Design review of the part built by this model. Coordinates are the model's own, in mm. A direction names the side the tool comes from. Round coordinates to 2 decimals unless told otherwise and drop trailing zeros. Write each loop counter-clockwise with the first axis right and the second up, starting at its lowest first coordinate (ties: lowest second). Pieces come first, ordered by that corner, then holes. Notation, with made-up numbers: (44.25, 16.5) -> (97.25, 16.5) arc R20 cw to (97.25, 20.5) -> close; hole circle Ø10 at (4, 86.25). An arc over 180 degrees is marked (long way). Write item = value, one per line. Start each with the question number.
Item 1: Add section A-A, the plane z = -13.5. State the section outline as (x, y) points, then the cut area to 3 significant figures.
Item 2: For pin 1 Ø17 at (x, z) = (123.5, -13.5) entering from -Y; pin 2 Ø2 at (x, z) = (120, -16.5) entering from -Y; pin 3 Ø4 at (x, z) = (121.5, -12.5) entering from -Y, all flat-tipped, find the tip position at first contact; note any pin that passes through.
Item 3: Add section C-C, the plane z = -3.5. State the section outline as (x, y) points.
Item 4: Add section B-B, the plane y = 2.45. State the section outline as (x, z) points, then the cut area to 3 significant figures.
Item 5: Mouldability with a two-part tool opening along X and no side actions: class faces 3 (the flat face through (59, 3, 1.5)), 4 (the cylindrical face through (-21.496, 2.958, -13.17)), 5 (the cylindrical face through (125, 4.99, -8.73)), 6 (the cylindrical face through (138.496, 2.958, -13.83)) as released by +X, released by -X, zero draft, split by the parting line, or undercut.
Item 6: To check wall thickness, follow L1, parallel to X at y = 1.3, z = -13.5; L2, parallel to X at y = 4.7, z = -13.5; L3, parallel to Z at x = -6.5, y = 5.1. State the ranges of each line that lie inside material, in increasing order.
Item 7: Add section D-D, the plane z = -24.5. State the section outline as (x, y) points, then the cut area to 3 significant figures.
Item 8: Machinability: for faces 1 (the flat face through (58, 3, -28.5)), 2 (the cylindrical face through (129.945, 1.972, -12.654)), which of the approach directions +Z, -Z, +X, -X, +Y, -Y give a long, thin tool a straight path to every point of the face, cutting with its end or side? Answer none if there is none.
from build123d import *

# Parameters (mm, degrees)
SKETCH2_R           = 5
BOSS_EXTRUDE1_DEPTH = 6
SKETCH4_R           = 6.5
CUT_EXTRUDE1_DEPTH  = 4


with BuildPart() as part:
    # Sketch2 → Boss-Extrude1 (new body)
    with BuildSketch(Plane(origin=(0, 0, 0), x_dir=(1, 0, 0), z_dir=(0, 1, 0))):
        with BuildLine():
            Line((-6.5, 28.5), (123.5, 28.5))
            ThreePointArc((123.5, 28.5), (138.5, 13.5), (123.5, -1.5))
            Line((123.5, -1.5), (-6.5, -1.5))
            ThreePointArc((-6.5, -1.5), (-21.5, 13.5), (-6.5, 28.5))
        make_face()
        with Locations(Location((-6.5, 13.5, 0), (0, 0, 270))):
            Circle(SKETCH2_R, mode=Mode.SUBTRACT)
        with Locations(Location((123.5, 13.5, 0), (0, 0, 270))):
            Circle(SKETCH2_R, mode=Mode.SUBTRACT)
    extrude(amount=BOSS_EXTRUDE1_DEPTH)

    # Sketch4 → Cut-Extrude1 (cut)
    with BuildSketch(Plane.XZ):
        with Locations(Location((123.5, -13.5, 0), (0, 0, 270))):
            Circle(SKETCH4_R)
        with Locations(Location((-6.5, -13.5, 0), (0, 0, 270))):
            Circle(SKETCH4_R)
    extrude(amount=-CUT_EXTRUDE1_DEPTH, mode=Mode.SUBTRACT)


solid = part.part
Result set:
q1.outline = (-21.5, 0) -> (-13, 0) -> (-13, 4) -> (-11.5, 4) -> (-11.5, 6) -> (-21.5, 6) -> close; (-1.5, 4) -> (0, 4) -> (0, 0) -> (117, 0) -> (117, 4) -> (118.5, 4) -> (118.5, 6) -> (-1.5, 6) -> close; (128.5, 4) -> (130, 4) -> (130, 0) -> (138.5, 0) -> (138.5, 6) -> (128.5, 6) -> close
q1.area = 816 mm²
q2.pin_1 = 0
q2.pin_2 = 4
q2.pin_3 = through
q3.outline = (-17.68, 0) -> (134.68, 0) -> (134.68, 6) -> (-17.68, 6) -> close
q4.outline = (-6.5, -28.5) -> (123.5, -28.5) arc R15 ccw to (123.5, 1.5) -> (-6.5, 1.5) arc R15 ccw to start; hole circle Ø13 at (-6.5, -13.5); hole circle Ø13 at (123.5, -13.5)
q4.area = 4,340 mm²
q5.face_3 = zero draft
q5.face_4 = released by -X
q5.face_5 = undercut
q5.face_6 = released by +X
q6.L1 = -21.5 to -13, 0 to 117, 130 to 138.5
q6.L2 = -21.5 to -11.5, -1.5 to 118.5, 128.5 to 138.5
q6.L3 = -28.5 to -18.5, -8.5 to 1.5
q7.outline = (-16.7, 0) -> (133.7, 0) -> (133.7, 6) -> (-16.7, 6) -> close
q7.area = 902 mm²
q8.face_1 = -Z, +X, -X, +Y, -Y
q8.face_2 = -Y
